from build123d import *

# Parameters (mm, degrees)
F1_DEPTH = 25.4
F2_DEPTH = 25.4


with BuildPart() as f1:
    # F0 (on Front) → F1 (new body)
    with BuildSketch(Plane.XZ):
        with BuildLine():
            Line((-29.6519356012, 52.650562261), (-29.6519356012, 0))
            Line((-29.6519356012, 0), (-29.6519356012, -52.650562261))
            ThreePointArc((-29.6519356012, -52.650562261), (-28.9342502123, -55.5830581471), (-26.9434215471, -57.8526849149))
            Line((-26.9434215471, -57.8526849149), (-1.1631480992, -75.8988767652))
            ThreePointArc((-1.1631480992, -75.8988767652), (5.4108337328, -76.3290687224), (8.8283378467, -70.6967541113))
            Line((8.8283378467, -70.6967541113), (8.8283378467, -37.4758915701))
            ThreePointArc((8.8283378467, -37.4758915701), (9.2975107187, -35.0804015806), (10.6356991979, -33.0388955022))
            Line((10.6356991979, -33.0388955022), (24.9684960825, -18.364842139))
            ThreePointArc((24.9684960825, -18.364842139), (26.3066845617, -16.3233360606), (26.7758574337, -13.9278460711))
            Line((26.7758574337, -13.9278460711), (26.7758574337, 0))
            Line((26.7758574337, 0), (26.7758574337, 13.9278460711))
            ThreePointArc((26.7758574337, 13.9278460711), (26.3066845617, 16.3233360606), (24.9684960825, 18.364842139))
            Line((24.9684960825, 18.364842139), (10.6356991979, 33.0388955022))
            ThreePointArc((10.6356991979, 33.0388955022), (9.2975107187, 35.0804015806), (8.8283378467, 37.4758915701))
            Line((8.8283378467, 37.4758915701), (8.8283378467, 70.6967541113))
            ThreePointArc((8.8283378467, 70.6967541113), (5.4108337328, 76.3290687224), (-1.1631480992, 75.8988767652))
            Line((-1.1631480992, 75.8988767652), (-26.9434215471, 57.8526849149))
            ThreePointArc((-26.9434215471, 57.8526849149), (-28.9342502123, 55.5830581471), (-29.6519356012, 52.650562261))
        make_face()
    extrude(amount=F1_DEPTH)

    # F2 (add): a face of the model
    f2_faces = [f1.faces().sort_by_distance(p)[0] for p in [
        (-5.4722080817, -25.4, 0),
    ]]
    extrude(f2_faces, amount=F2_DEPTH)


solid = f1.part
Design review of the part built by this model. Coordinates are the model's own, in mm. A direction names the side the tool comes from. Round coordinates to 2 decimals unless told otherwise and drop trailing zeros. Loops run counter-clockwise (first coordinate to the right, second up) from the corner with the lowest first, then second, coordinate; pieces in that order, holes last. Notation, with made-up numbers: (6.5, 33.5) -> (20.5, 33.5) arc R28 cw to (20.5, 52.5) -> close; hole circle Ø2 at (3.25, -20). An arc over 180 degrees is marked (long way). Use one line per item in the form item = value. Start each with the question number.
Q1. For pin 1 Ø4 at (x, y) = (14.5, -26) entering from -Z; pin 2 Ø1 at (x, y) = (7, -12) entering from -Z; pin 3 Ø5 at (x, y) = (13, -22.5) entering from +Z, all flat-tipped, find the tip position at first contact; note any pin that passes through.
Q2. We need section B-B on z = -41. Give the boundary of the cut face in (x, y), then the cut area to 3 significant figures.
Q3. We need section C-C on x = 7. Give the boundary of the cut face in (y, z).
Q4. Machinability: for faces 1 (the face through (-28.95, -25.04, -55.55)), 2 (the face through (8.828, -25, 54)), 3 (the face through (8.828, -25, -54)), which of the approach directions +Z, -Z, +X, -X, +Y, -Y give a long, thin tool a straight path to every point of the face, cutting with its end or side? Answer none if there is none.
Q5. We need section A-A on y = -15. Give the boundary of the cut face in (x, z), then the cut area to 3 significant figures.
Q6. Wall thickness on line 1 along X through (y, z) = (-29.5, -41); line 2 along Z through (x, y) = (-19, -32); line 3 along X through (y, z) = (-40, -16): over which ranges is each line inside the solid? List them lowest first. Write a range as [from, to].
Calculated:
q1.pin_1 = -31.13
q1.pin_2 = -75.61
q1.pin_3 = 33.18
q2.outline = (-29.65, -50.8) -> (8.83, -50.8) -> (8.83, 0) -> (-29.65, 0) -> close
q2.area = 1,950 mm²
q3.outline = (-50.8, -75.16) -> (0, -75.16) -> (0, 75.16) -> (-50.8, 75.16) -> close
q4.face_1 = -Z, -X, +Y, -Y
q4.face_2 = +Z, +X, +Y, -Y
q4.face_3 = -Z, +X, +Y, -Y
q5.outline = (-29.65, -52.65) arc R6.35 ccw to (-26.94, -57.85) -> (-1.16, -75.9) arc R6.35 ccw to (8.83, -70.7) -> (8.83, -37.48) arc R6.35 cw to (10.64, -33.04) -> (24.97, -18.36) arc R6.35 ccw to (26.78, -13.93) -> (26.78, 13.93) arc R6.35 ccw to (24.97, 18.36) -> (10.64, 33.04) arc R6.35 cw to (8.83, 37.48) -> (8.83, 70.7) arc R6.35 ccw to (-1.16, 75.9) -> (-26.94, 57.85) arc R6.35 ccw to (-29.65, 52.65) -> close
q5.area = 6,200 mm²
q6.line_1 = [-29.65, 8.83]
q6.line_2 = [-63.41, 63.41]
q6.line_3 = [-29.65, 26.43]
